Read the model definition and answer for the solid it produces. Units are mm, in the model's axes. A direction names the side the tool comes from. Round coordinates to 2 decimals unless told otherwise and drop trailing zeros. Loops run counter-clockwise (first coordinate to the right, second up) from the corner with the lowest first, then second, coordinate; pieces in that order, holes last. Notation, with made-up numbers: (-23.5, 6) -> (-12.5, 6) arc R28 ccw to (-12.5, 36) -> close; hole circle Ø6 at (18, 83.25). An arc over 180 degrees is marked (long way). Put each result on its own line as item: value.
from build123d import *

# Parameters (mm, degrees)
F0_R        = 10.5
F0_R_2      = 1.375
F0_W        = 14.5
F0_H        = 14.06
F1_DEPTH    = 24
F2_T        = 2
F2_T3_DEPTH = 28
F0_R_3      = 9.5
F3_DEPTH    = 30
F0_R_4      = 1
F4_DEPTH    = 2
F5_R        = 1
F6_R        = 3.375
F7_DEPTH    = 22
F9_DEPTH    = 22
F10_W       = 10.5
F10_H       = 11.5
F11_DEPTH   = 2


# Not quite as in the source:
# - an extrude ends at something that could not be found from the text; its depth is read off the source's solid
# - a shell that OpenCascade refuses in one call is made with other operations: the cavity is built on its own and cut out


with BuildPart() as f1:
    # F0 (on Front) → F1 (new body)
    with BuildSketch(Plane.XZ):
        Polygon((-7.25, 32.5), (-13.7, 32.5), (-13.7, 7.4914984291), (-13.7, -14.5085015709), (-13.7, -32.5), (13.7, -32.5), (13.7, -14.5420665913), (13.7, 7.4579334087), (13.7, 32.5), (7.25, 32.5), align=None)
        with Locations((0, -4.91)):
            Circle(F0_R, mode=Mode.SUBTRACT)
        with Locations((6.2, 10.09)):
            Circle(F0_R_2, mode=Mode.SUBTRACT)
        with Locations((0, 39.53)):
            Rectangle(F0_W, F0_H)
    extrude(amount=F1_DEPTH)

    # F2: shell of thickness 2, made by hand


with BuildPart() as f2_core1:
    # F2_t2: copy of F1
    add(f1.part)

    # the walls: a layer under each face that stays
    f2_faces = [f2_core1.faces().sort_by_distance(p)[0] for p in [
        (-10.475, -12, 32.5),
        (-13.7, -12, 0),
        (0, -12, -32.5),
        (13.7, -12, 0),
        (10.475, -12, 32.5),
        (7.25, -12, 39.53),
        (0, -12, 46.56),
        (-7.25, -12, 39.53),
        (-10.5, -12, -4.91),
        (4.825, -12, 10.09),
        (0, -24, 7.03),
    ]]
    thicken(f2_faces, amount=-F2_T, mode=Mode.SUBTRACT)

    # F2_s4 → F2_t3 (cut)
    with BuildSketch(Plane.XZ.offset(-2)):
        Polygon((-7.27, 32.52), (-7.25, 30.5), (-5.25, 30.5), (-5.25, 32.5), align=None)
        Polygon((7.27, 32.52), (7.25, 30.5), (5.25, 30.5), (5.25, 32.5), align=None)
    extrude(amount=F2_T3_DEPTH, mode=Mode.SUBTRACT)


with BuildPart() as f1_1:
    add(f1.part)

    # what is left inside the walls is the cavity
    f2_cavity = [f2_core1.part.solids().sort_by_distance(p)[0] for p in [
        (0, -0.02, 14.513333),
        (0, -14.666667, -17.43),
    ]]
    add(f2_cavity, mode=Mode.SUBTRACT)

    # F0 (on Front) → F3 (join)
    with BuildSketch(Plane.XZ):
        with Locations((0, -4.91)):
            Circle(F0_R)
        with Locations((0, -4.91)):
            Circle(F0_R_3, mode=Mode.SUBTRACT)
    extrude(amount=F3_DEPTH)

    # F0 (on Front) → F4 (join)
    with BuildSketch(Plane.XZ):
        with BuildLine():
            Line((-13.7, -14.5085015709), (-13.7, 7.4914984291))
            add(Edge.make_bspline(
                [(-19.093351697, -3.5085015709), (-19.1026122295, 2.6293974578), (-13.7, -0.8116166133), (-13.7, 7.4914984291)],
                knots=[0, 0, 0, 0, 12.2510506704, 12.2510506704, 12.2510506704, 12.2510506704], degree=3))
            add(Edge.make_bspline(
                [(-19.093351697, -3.5085015709), (-19.0674920552, -9.0708802246), (-13.7, -6.7231292221), (-13.7, -14.5085015709)],
                knots=[0, 0, 0, 0, 12.2510506704, 12.2510506704, 12.2510506704, 12.2510506704], degree=3))
        make_face()
        with Locations((-16, -3.5420665913)):
            Circle(F0_R_4, mode=Mode.SUBTRACT)
        with BuildLine():
            add(Edge.make_bspline(
                [(19.0999998349, -3.5410547692), (19.0290823921, 2.4940823569), (13.7, -0.9160112299), (13.7, 7.4579334087)],
                knots=[0, 0, 0, 0, 12.2530706011, 12.2530706011, 12.2530706011, 12.2530706011], degree=3))
            Line((13.7, 7.4579334087), (13.7, -14.5420665913))
            add(Edge.make_bspline(
                [(19.0999998349, -3.5410547692), (19.0287452534, -10.2770104641), (13.7, -7.3807572052), (13.7, -14.5420665913)],
                knots=[0, 0, 0, 0, 12.2548871608, 12.2548871608, 12.2548871608, 12.2548871608], degree=3))
        make_face()
        with Locations((16, -3.5420665913)):
            Circle(F0_R_4, mode=Mode.SUBTRACT)
    extrude(amount=F4_DEPTH)

    # F5
    f5_edges = [f1_1.edges().sort_by_distance(p)[0] for p in [
        (13.7, -12, 32.5),
        (-13.7, -12, 32.5),
        (-13.7, -12, -32.5),
        (13.7, -12, -32.5),
        (7.25, -12, 46.56),
        (-7.25, -12, 46.56),
        (7.25, -24, 39.53),
        (-7.25, -24, 39.53),
        (-13.7, -24, 0),
        (13.7, -24, 0),
        (0, -24, -32.5),
        (-10.475, -24, 32.5),
        (10.475, -24, 32.5),
        (0, -24, 46.56),
    ]]
    fillet(f5_edges, radius=F5_R)

    # F6 (on face) → F7 (cut, through all)
    with BuildSketch(Plane(origin=(0, 0, 0), x_dir=(-1, 0, 0), z_dir=(0, 1, 0))):
        with Locations((-6.2, 10.09)):
            Circle(F6_R)
    extrude(amount=-F7_DEPTH, mode=Mode.SUBTRACT)

    # F8 (on face) → F9 (cut, through all)
    with BuildSketch(Plane(origin=(0, 0, 0), x_dir=(-1, 0, 0), z_dir=(0, 1, 0))):
        with BuildLine():
            ThreePointArc((-11.7, -9.31), (0, -17.41), (11.7, -9.31))
            Line((11.7, -9.31), (11.7, -0.51))
            ThreePointArc((11.7, -0.51), (0, 7.59), (-11.7, -0.51))
            Line((-11.7, -0.51), (-11.7, -9.31))
        make_face()
    extrude(amount=-F9_DEPTH, mode=Mode.SUBTRACT)

    # F10 (on face) → F11 (cut, through all)
    with BuildSketch(Plane.YZ.offset(13.7)):
        with Locations((-5.25, 13.6579334087)):
            Rectangle(F10_W, F10_H)
    extrude(amount=-F11_DEPTH, mode=Mode.SUBTRACT)


solid = f1_1.part
Item 1: The part is cut by section A-A (x = 0). Determine the outline of the cut face in (y, z), then the cut area to 3 significant figures.
Derived:
outline: (-30, -15.41) -> (-24, -15.41) -> (-24, -31.5) arc R1 ccw to (-23, -32.5) -> (0, -32.5) -> (0, -30.5) -> (-22, -30.5) -> (-22, -14.41) -> (-30, -14.41) -> close; (-30, 4.59) -> (-22, 4.59) -> (-22, 44.56) -> (0, 44.56) -> (0, 46.56) -> (-23, 46.56) arc R1 ccw to (-24, 45.56) -> (-24, 5.59) -> (-30, 5.59) -> close
area: 220 mm^2
Item 2: The part is cut by section B-B (z = 10.09). Determine the outline of the cut face in (x, y) (3 decimals), then the cut area to 3 significant figures.
Derived:
outline: (-13.7, -23) arc R1 ccw to (-12.7, -24) -> (4.825, -24) -> (4.825, -22) -> (-11.7, -22) -> (-11.7, 0) -> (-13.7, 0) -> close; (7.575, -24) -> (12.7, -24) arc R1 ccw to (13.7, -23) -> (13.7, -10.5) -> (11.7, -10.5) -> (11.7, -22) -> (7.575, -22) -> close
area: 116 mm^2
Item 3: Which of the six approach directions +Z, -Z, +X, -X, +Y, -Y give full straight-line access (tool end or side, diameter ignored) to faces 1 (the flat face through (10, -11, 32.5)), 2 (the flat face through (13, -5, 7.908)), 3 (the flat face through (-14.6, -2, -3.4)), 4 (the flat face through (-8, -11, 30.5)), 5 (the flat face through (-10, -11, 32.5))?
Derived:
face 1: +Z, +X, +Y, -Y
face 2: +X, +Y
face 3: +Z, -Z, -X, -Y
face 4: +Y
face 5: +Z, -X, +Y, -Y
Item 4: Find the intervals of material crossed by line 1 along X through (y, z) = (-23, 10); line 2 along Z through (x, y) = (6.2, -22.6) (3 decimals); line 3 along Z through (x, y) = (0, -24.75), in increasing order.
Derived:
line 1: x = -13.7 to 4.83, 7.57 to 13.7
line 2: z = -32.5 to -12.108, 2.288 to 8.715, 11.465 to 46.56
line 3: z = -15.41 to -14.41, 4.59 to 5.59
Item 5: The part is cut by section C-C (y = -11.5). Determine the outline of the cut face in (x, z).
Derived:
outline: (-13.7, -31.5) arc R1 ccw to (-12.7, -32.5) -> (12.7, -32.5) arc R1 ccw to (13.7, -31.5) -> (13.7, 31.5) arc R1 ccw to (12.7, 32.5) -> (7.25, 32.5) -> (7.25, 45.56) arc R1 ccw to (6.25, 46.56) -> (-6.25, 46.56) arc R1 ccw to (-7.25, 45.56) -> (-7.25, 32.5) -> (-12.7, 32.5) arc R1 ccw to (-13.7, 31.5) -> close; hole (-11.7, -30.5) -> (11.7, -30.5) -> (11.7, 30.5) -> (5.25, 30.5) -> (5.25, 44.56) -> (-5.25, 44.56) -> (-5.25, 30.5) -> (-11.7, 30.5) -> close
Item 6: Flat-ended cylindrical pins translate along their axes: pin 1 Ø4 at (y, z) = (-9, 36) entering from -X; pin 2 Ø0.6 at (x, z) = (12.5, 15.5) entering from +Y; pin 3 Ø6 at (y, z) = (-10.5, -19) entering from +X. Find the tip coordinate at first contact, or state that the pin passes through.
Derived:
pin 1: stops at x = -7.25
pin 2: stops at y = -10.5
pin 3: stops at x = 13.7
Item 7: The part is cut by section D-D (z = 23). Determine the outline of the cut face in (x, y).
Derived:
outline: (-13.7, -23) arc R1 ccw to (-12.7, -24) -> (12.7, -24) arc R1 ccw to (13.7, -23) -> (13.7, 0) -> (11.7, 0) -> (11.7, -22) -> (-11.7, -22) -> (-11.7, 0) -> (-13.7, 0) -> close
